Can you work these out from the drawing? Everything is in mm from the part's minimum corner. A direction names the side the tool comes from. Coordinates: 2 decimals unless noted, no trailing zeros. Order: outer loops, then holes, each group sorted by start corner. A loop starts at its lowest first (then second) coordinate and runs counter-clockwise, first axis right, second up. Notation, with made-up numbers: (63.25, 25.5) - (99.25, 25.5) arc R15 cw to (99.25, 53.5) - close; hole circle Ø10 at (30.5, 17). An arc over 180 degrees is marked (long way). One line per item, written item: value.
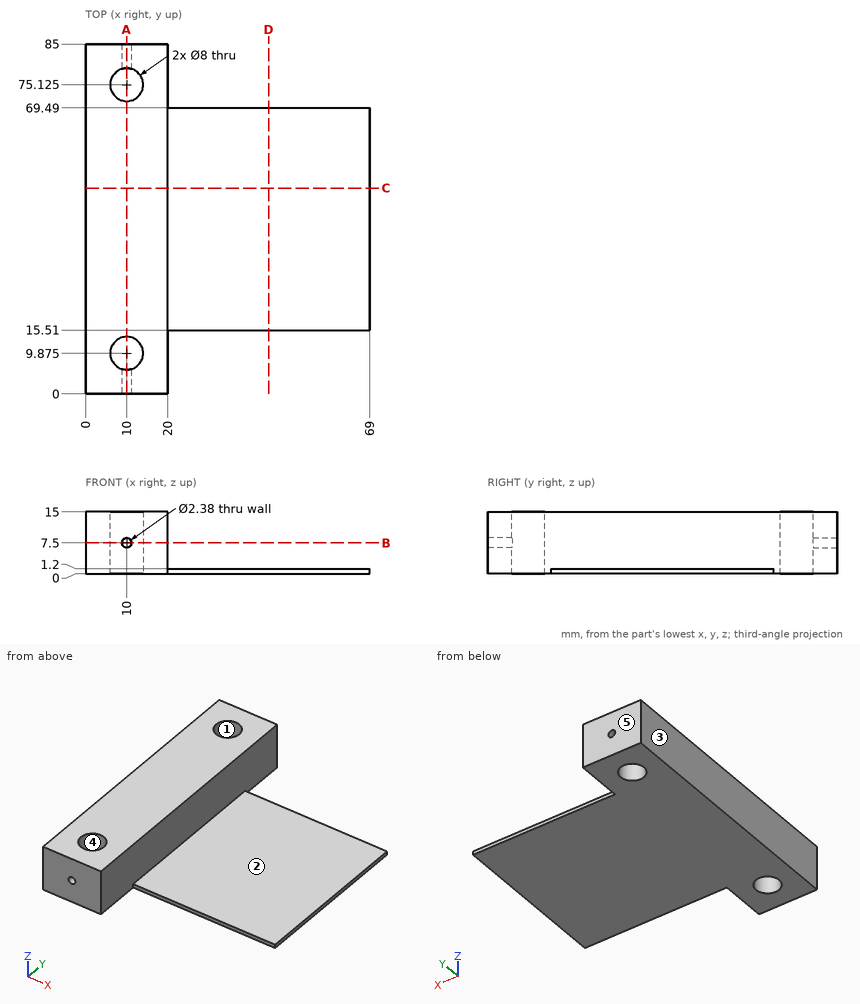
Item 1: I want a section at B-B on z = 7.5. Please give me the cut outline in (x, y) (3 decimals).
Conclusion:
outline: (0, 0) - (8.81, 0) - (8.81, 6.056) arc R4 cw (long way) to (11.19, 6.056) - (11.19, 0) - (20, 0) - (20, 85) - (11.19, 85) - (11.19, 78.944) arc R4 cw (long way) to (8.81, 78.944) - (8.81, 85) - (0, 85) - close
Item 2: Thinking about a two-plate mould opening in X: for the marked faces 3, 4 and 5, which applies, pulls with the +X half, pulls with the -X half, needs draft (parallel to the pull), parting line crosses it, or undercut?
Conclusion:
face 3: pulls with the -X half
face 4: undercut
face 5: needs draft
Item 3: If I drill on probe 1 along Y at (x, z) = (10, 5) (3 decimals); probe 2 along Z at (x, y) = (10, 4); probe 3 along Y at (x, z) = (6.5, 1.25), over which ranges is the centre line in solid material (lowest first)?
Conclusion:
probe 1: 0 to 5.875, 13.875 to 71.125, 79.125 to 85
probe 2: 0 to 6.31, 8.69 to 15
probe 3: 0 to 7.94, 11.81 to 73.19, 77.06 to 85
Item 4: I'm going to push flat-ended pins straight in: pin 1 Ø1.4 at (x, z) = (10, 7.5) entering from +Y; pin 2 Ø6.5 at (x, y) = (10, 75.125) entering from -Z; pin 3 Ø6 at (x, y) = (40, 55.5) entering from +Z; pin 4 Ø0.6 at (x, z) = (38, 0.5) entering from -Y. Where does each tip first touch, or does it pass through?
Conclusion:
pin 1: y = 71.19
pin 2: through
pin 3: z = 1.2
pin 4: y = 15.51
Item 5: I want a section at D-D on x = 44.5. Please give me the cut outline in (y, z), then the cut area to 3 significant figures.
Conclusion:
outline: (15.51, 0) - (69.49, 0) - (69.49, 1.2) - (15.51, 1.2) - close
area: 64.8 mm²
Item 6: For the marked faces 1 and 2, which set-ups out of +Z, -Z, +X, -X, +Y, -Y let a thin tool reach every point of the face, with its end or its side?
Conclusion:
face 1: +Z, -Z
face 2: +Z, +X, +Y, -Y
Item 7: I want a section at C-C on y = 50. Please give me the cut outline in (x, z), then the cut area to 3 significant figures.
Conclusion:
outline: (0, 0) - (69, 0) - (69, 1.2) - (20, 1.2) - (20, 15) - (0, 15) - close
area: 359 mm²
Item 8: I want a section at A-A on x = 10. Please give me the cut outline in (y, z) (3 decimals).
Conclusion:
outline: (0, 0) - (5.875, 0) - (5.875, 6.31) - (0, 6.31) - close; (0, 8.69) - (5.875, 8.69) - (5.875, 15) - (0, 15) - close; (13.875, 0) - (71.125, 0) - (71.125, 15) - (13.875, 15) - close; (79.125, 0) - (85, 0) - (85, 6.31) - (79.125, 6.31) - close; (79.125, 8.69) - (85, 8.69) - (85, 15) - (79.125, 15) - close
